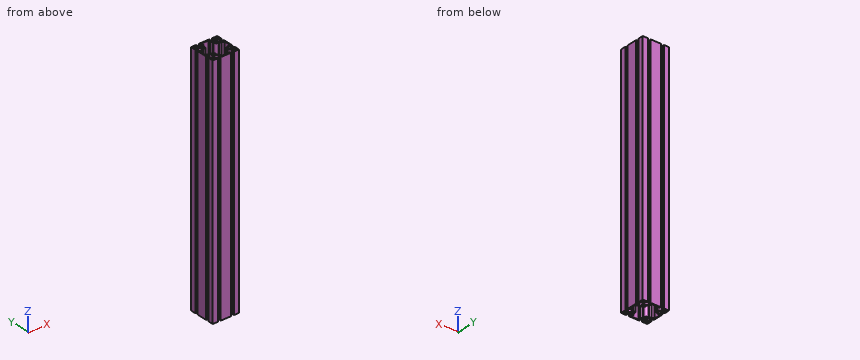
```python
from build123d import *

# Parameters (mm, degrees)
SKETCH_1_R      = 3.4
SKETCH_1_R_2    = 4
EXTRUDE_1_DEPTH = 360


with BuildPart() as part:
    # 草图1 → 凸台-拉伸1 (new, symmetric)
    with BuildSketch(Plane.XY):
        with BuildLine():
            Line((-40, 40), (-24.25, 40))
            Line((-24.25, 40), (-24.25, 36))
            Line((-24.25, 36), (-27.15, 36))
            Line((-27.15, 36), (-27.15, 29))
            ThreePointArc((-27.15, 29), (-20, 25.5), (-12.85, 29))
            Line((-12.85, 29), (-12.85, 36))
            Line((-12.85, 36), (-15.75, 36))
            Line((-15.75, 36), (-15.75, 40))
            Line((-15.75, 40), (15.75, 40))
            Line((15.75, 40), (15.75, 36))
            Line((15.75, 36), (12.85, 36))
            Line((12.85, 36), (12.85, 29))
            ThreePointArc((12.85, 29), (20, 25.5), (27.15, 29))
            Line((27.15, 29), (27.15, 36))
            Line((27.15, 36), (24.25, 36))
            Line((24.25, 36), (24.25, 40))
            Line((24.25, 40), (40, 40))
            Line((40, 40), (40, 24.25))
            Line((40, 24.25), (36, 24.25))
            Line((36, 24.25), (36, 27.15))
            Line((36, 27.15), (29, 27.15))
            ThreePointArc((29, 27.15), (25.5, 20), (29, 12.85))
            Line((29, 12.85), (36, 12.85))
            Line((36, 12.85), (36, 15.75))
            Line((36, 15.75), (40.000271684, 15.75))
            Line((40.000271684, 15.75), (40.000271684, -15.75))
            Line((40.000271684, -15.75), (36, -15.75))
            Line((36, -15.75), (36, -12.85))
            Line((36, -12.85), (29, -12.85))
            ThreePointArc((29, -12.85), (25.5, -20), (29, -27.15))
            Line((29, -27.15), (36, -27.15))
            Line((36, -27.15), (36, -24.25))
            Line((36, -24.25), (40, -24.25))
            Line((40, -24.25), (40, -40))
            Line((40, -40), (24.25, -40))
            Line((24.25, -40), (24.25, -36))
            Line((24.25, -36), (27.15, -36))
            Line((27.15, -36), (27.15, -29))
            ThreePointArc((27.15, -29), (20, -25.5), (12.85, -29))
            Line((12.85, -29), (12.85, -36))
            Line((12.85, -36), (15.75, -36))
            Line((15.75, -36), (15.75, -40))
            Line((15.75, -40), (-15.75, -40))
            Line((-15.75, -40), (-15.75, -36))
            Line((-15.75, -36), (-12.85, -36))
            Line((-12.85, -36), (-12.85, -29))
            ThreePointArc((-12.85, -29), (-20, -25.5), (-27.15, -29))
            Line((-27.15, -29), (-27.15, -36))
            Line((-27.15, -36), (-24.25, -36))
            Line((-24.25, -36), (-24.25, -40))
            Line((-24.25, -40), (-40, -40))
            Line((-40, -40), (-40, -24.25))
            Line((-40, -24.25), (-36, -24.25))
            Line((-36, -24.25), (-36, -27.15))
            Line((-36, -27.15), (-29, -27.15))
            ThreePointArc((-29, -27.15), (-25.5, -20), (-29, -12.85))
            Line((-29, -12.85), (-36, -12.85))
            Line((-36, -12.85), (-36, -15.75))
            Line((-36, -15.75), (-40.000271684, -15.75))
            Line((-40.000271684, -15.75), (-40.000271684, 15.75))
            Line((-40.000271684, 15.75), (-36, 15.75))
            Line((-36, 15.75), (-36, 12.85))
            Line((-36, 12.85), (-29, 12.85))
            ThreePointArc((-29, 12.85), (-25.5, 20), (-29, 27.15))
            Line((-29, 27.15), (-36, 27.15))
            Line((-36, 27.15), (-36, 24.25))
            Line((-36, 24.25), (-40, 24.25))
            Line((-40, 24.25), (-40, 40))
        make_face()
        with Locations(Location((-20, 20, 0), (0, 0, 180))):
            Circle(SKETCH_1_R, mode=Mode.SUBTRACT)
        with Locations(Location((-33.575, 33.575, 0), (0, 0, 180))):
            Circle(SKETCH_1_R_2, mode=Mode.SUBTRACT)
        with Locations(Location((33.575, 33.575, 0), (0, 0, 180))):
            Circle(SKETCH_1_R_2, mode=Mode.SUBTRACT)
        with Locations(Location((20, 20, 0), (0, 0, 180))):
            Circle(SKETCH_1_R, mode=Mode.SUBTRACT)
        with Locations(Location((20, -20, 0), (0, 0, 180))):
            Circle(SKETCH_1_R, mode=Mode.SUBTRACT)
        with Locations(Location((33.575, -33.575, 0), (0, 0, 180))):
            Circle(SKETCH_1_R_2, mode=Mode.SUBTRACT)
        with Locations(Location((-33.575, -33.575, 0), (0, 0, 180))):
            Circle(SKETCH_1_R_2, mode=Mode.SUBTRACT)
        with Locations(Location((-20, -20, 0), (0, 0, 180))):
            Circle(SKETCH_1_R, mode=Mode.SUBTRACT)
        with BuildLine():
            Line((10.35, 37), (-10.35, 37))
            Line((-10.35, 37), (-10.35, 29))
            Line((-10.35, 29), (-14.5, 24.85))
            Line((-14.5, 24.85), (-14.5, 20))
            ThreePointArc((-14.5, 20), (-16.110912703, 16.110912703), (-20, 14.5))
            Line((-20, 14.5), (-24.85, 14.5))
            Line((-24.85, 14.5), (-29, 10.35))
            Line((-29, 10.35), (-37, 10.35))
            Line((-37, 10.35), (-37, -10.35))
            Line((-37, -10.35), (-29, -10.35))
            Line((-29, -10.35), (-24.85, -14.5))
            Line((-24.85, -14.5), (-20, -14.5))
            ThreePointArc((-20, -14.5), (-16.110912703, -16.110912703), (-14.5, -20))
            Line((-14.5, -20), (-14.5, -24.85))
            Line((-14.5, -24.85), (-10.35, -29))
            Line((-10.35, -29), (-10.35, -37))
            Line((-10.35, -37), (10.35, -37))
            Line((10.35, -37), (10.35, -29))
            Line((10.35, -29), (14.5, -24.85))
            Line((14.5, -24.85), (14.5, -20))
            ThreePointArc((14.5, -20), (16.110912703, -16.110912703), (20, -14.5))
            Line((20, -14.5), (24.85, -14.5))
            Line((24.85, -14.5), (29, -10.35))
            Line((29, -10.35), (37, -10.35))
            Line((37, -10.35), (37, 10.35))
            Line((37, 10.35), (29, 10.35))
            Line((29, 10.35), (24.85, 14.5))
            Line((24.85, 14.5), (20, 14.5))
            ThreePointArc((20, 14.5), (16.110912703, 16.110912703), (14.5, 20))
            Line((14.5, 20), (14.5, 24.85))
            Line((14.5, 24.85), (10.35, 29))
            Line((10.35, 29), (10.35, 37))
        make_face(mode=Mode.SUBTRACT)
    extrude(amount=EXTRUDE_1_DEPTH, both=True)


solid = part.part
```
Verification items for the finished model (mm, model axes). Give positions to 0.01 mm unless a question says otherwise; leave off trailing zeros. Order: outer loops, then holes, each group sorted by start corner. A loop starts at its lowest first (then second) coordinate and runs counter-clockwise, first axis right, second up. Notation, with made-up numbers: (58, -11.75) - (107, -11.75) arc R24 cw to (107, 9.25) - close; hole circle Ø6 at (48, 57). An arc over 180 degrees is marked (long way). Answer as CSV lines item,"result". Start each with the question number.
Item 1: Gauge pin test, flat ends, axial feed: pin 1 (1 mm diameter, centred on y = 18.5, z = -251.5, fed in from +X); pin 2 (2.5 mm diameter, centred on x = 21.5, z = 18, fed in from +Y); pin 3 (4 mm diameter, centred on y = 22, z = 81.5, fed in from -X). Record the tip position at first contact, or that the pin passes through.
Item 2: Section check C-C, the plane z = 297.5. State how many separate pieces and enclosed holes the cut face has, plus the area to 3 significant figures.
Item 3: Section check A-A, the plane x = -2. Record the boundary of the cut face in (y, z).
Item 4: Material ranges on L1, parallel to Y at x = -20, z = 24; L2, parallel to X at y = 33.5, z = 259, recorded low to high.
Filled in:
1,pin 1,"x = 25.72"
1,pin 2,"y = 25.93"
1,pin 3,"x = -26.43"
2,separate pieces,"1"
2,enclosed holes,"9"
2,area,"1,560 mm^2"
3,outline,"(-40, -360) - (-37, -360) - (-37, 360) - (-40, 360) - close; (37, -360) - (40, -360) - (40, 360) - (37, 360) - close"
4,L1,"-25.5 to -23.4, -16.6 to -14.5, 14.5 to 16.6, 23.4 to 25.5"
4,L2,"-40 to -37.57, -29.58 to -27.15, -12.85 to -10.35, 10.35 to 12.85, 27.15 to 29.58, 37.57 to 40"
